```python
from build123d import *

# Parameters (mm, degrees)
SKETCH1_W           = 10
SKETCH1_H           = 5
EXTRUDE1_DEPTH      = 2.30625
SKETCH2_R           = 1.4224
EXTRUDE2_DEPTH      = 11
BOSS_EXTRUDE1_DEPTH = 4.6125


with BuildPart() as part:
    # Sketch1 → Extrude1 (new body, symmetric)
    with BuildSketch(Plane.XY):
        with Locations((-5, 0)):
            Rectangle(SKETCH1_W, SKETCH1_H)
    extrude(amount=EXTRUDE1_DEPTH, both=True)

    # Sketch2 → Extrude2 (cut, through all)
    with BuildSketch(Plane(origin=(0, 0, 0), x_dir=(0, 0, -1), z_dir=(1, 0, 0))):
        Circle(SKETCH2_R)
    extrude(amount=-EXTRUDE2_DEPTH, mode=Mode.SUBTRACT)

    # Sketch3 → Boss-Extrude1 (add)
    with BuildSketch(Plane(origin=(0, 0, -2.30625), x_dir=(-1, 0, 0), z_dir=(0, 0, -1))):
        with BuildLine():
            Line((10, 57.382622929), (10, 2.5))
            Line((10, 2.5), (0, 2.5))
            Line((0, 2.5), (0, 57.7))
            ThreePointArc((0, 57.7), (5.002517571, 57.620635762), (10, 57.382622929))
        make_face()
        with BuildLine():
            Line((0, -54.725), (0, -2.5))
            Line((0, -2.5), (10, -2.5))
            Line((10, -2.5), (10, -55.843170121))
            ThreePointArc((10, -55.843170121), (5.031160513, -55.005410893), (0, -54.725))
        make_face()
    extrude(amount=-BOSS_EXTRUDE1_DEPTH)


solid = part.part
```
Geometry check sheet. Reference: the model listing, model coordinates, mm. Round coordinates to 2 decimals unless told otherwise and drop trailing zeros. Order: outer loops, then holes, each group sorted by start corner. A loop starts at its lowest first (then second) coordinate and runs counter-clockwise, first axis right, second up. Notation, with made-up numbers: (-36.5, -35.75) -> (-24.5, -35.75) arc R28 ccw to (-24.5, -12.75) -> close; hole circle Ø5 at (33.5, 24). An arc over 180 degrees is marked (long way). Return JSON: item names as keys, results as strings. Group by question number.
Q1. Gauge pin test, flat end, axial feed: pin 1 (2.5 mm diameter, centred on y = 0, z = 0, fed in from -X). Record the tip position at first contact, or that the pin passes through.
Q2. Section check B-B, the plane z = 0. Record the boundary of the cut face in (x, y) (3 decimals).
Q3. Material ranges on probe 1 along Y at (x, z) = (-6.5, 0); probe 2 along Y at (x, z) = (-7.5, 0); probe 3 along Y at (x, z) = (-0.5, 1.8), recorded low to high. Write a range as from..to.
Q4. Release check for a two-part mould opening along Z. For faces 1 (the flat face through (0, 1, -2)), 2 (the cylindrical face through (-4.93, -1.39, 0.31)), 3 (the flat face through (-5, 2, -2.306)), 4 (the flat face through (-5, 2, 2.306)) record: released by +Z, released by -Z, zero draft, split by the parting line, or undercut.
Q5. Section check A-A, the plane y = 0. Record the boundary of the cut face in (x, z).
Q6. Section check C-C, the plane x = -6. Record the boundary of the cut face in (y, z), plus the area to 3 significant figures.
Numbers:
{
 "1": {"pin 1": "through"},
 "2": {"outline": "(-10, -55.843) arc R45.275 cw to (0, -54.725) -> (0, -1.422) -> (-10, -1.422) -> close; (-10, 1.422) -> (0, 1.422) -> (0, 57.7) arc R157.7 ccw to (-10, 57.383) -> close"},
 "3": {"probe 1": "-55.19..-1.42, 1.42..57.57", "probe 2": "-55.35..-1.42, 1.42..57.52", "probe 3": "-54.73..57.7"},
 "4": {"face 1": "zero draft", "face 2": "undercut", "face 3": "released by -Z", "face 4": "released by +Z"},
 "5": {"outline": "(-10, -2.31) -> (0, -2.31) -> (0, -1.42) -> (-10, -1.42) -> close; (-10, 1.42) -> (0, 1.42) -> (0, 2.31) -> (-10, 2.31) -> close"},
 "6": {"outline": "(-55.12, -2.31) -> (57.59, -2.31) -> (57.59, 2.31) -> (-55.12, 2.31) -> close; hole circle Ø2.84 at (0, 0)", "area": "514 mm^2"}
}
